Geometry: see drawing. Coordinates: mm, zero at the bounding-box minimum. A direction names the side the tool comes from. Give positions to 0.01 mm unless a question says otherwise; leave off trailing zeros. Loops run counter-clockwise (first coordinate to the right, second up) from the corner with the lowest first, then second, coordinate; pieces in that order, holes last. Notation, with made-up numbers: (-2, -5) - (45, -5) arc R14 ccw to (45, 8) - close; hole circle Ø2 at (-13, -28.75). An arc over 180 degrees is marked (long way). Use one line per item in the form item = value.
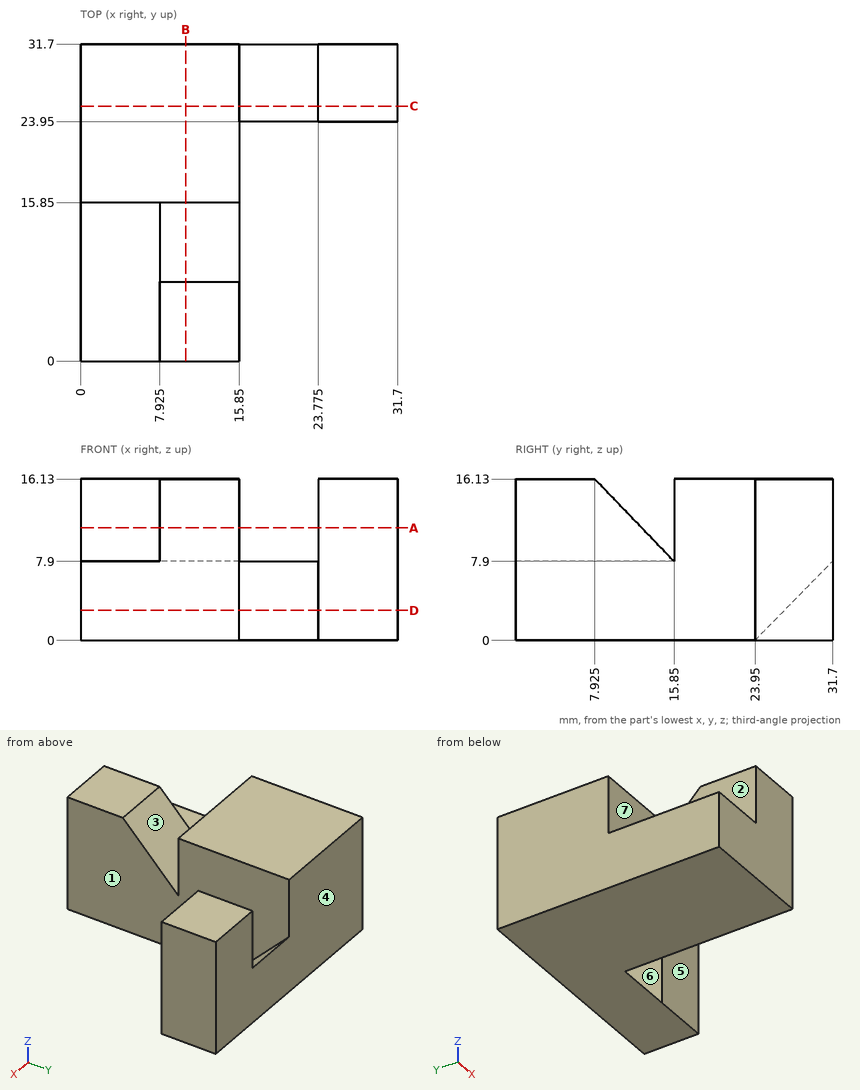
(1) Cut plane A-A (z = 11.25). Return the cut outline in (x, y) (3 decimals).
Solution:
outline = (0, 15.85) - (15.85, 15.85) - (15.85, 31.7) - (0, 31.7) - close; (7.925, 0) - (15.85, 0) - (15.85, 12.624) - (7.925, 12.624) - close; (23.775, 23.95) - (31.7, 23.95) - (31.7, 31.7) - (23.775, 31.7) - close
(2) Material intervals for L1, parallel to X at y = 24, z = 1.5 (3 decimals); L2, parallel to Y at x = 25, z = 8.5; L3, parallel to X at y = 22, z = 15.25, sorted ascending. Write a range as from..to.
Solution:
L1 = 0..15.85, 23.775..31.7
L2 = 23.95..31.7
L3 = 0..15.85
(3) Cut plane C-C (y = 25.5). Return the cut outline in (x, z) (3 decimals).
Solution:
outline = (0, 0) - (31.7, 0) - (31.7, 16.13) - (23.775, 16.13) - (23.775, 1.58) - (15.85, 1.58) - (15.85, 16.13) - (0, 16.13) - close
(4) Pin query (flat end, axial travel): P1, Ø4, axis at y = 12.5, z = 14, coming from the -X side (3 decimals); P2, Ø8, axis at y = 18.5, z = 5.5, coming from the +X side; P3, Ø4, axis at x = 28.5, z = 7.5, coming from the -Y side. Return the tip coordinate at first contact, or that it passes through.
Solution:
P1 = 7.925
P2 = 15.85
P3 = 23.95
(5) Cut plane B-B (x = 10.5). Return the cut outline in (y, z) (3 decimals), plus the area to 3 significant figures.
Solution:
outline = (0, 0) - (31.7, 0) - (31.7, 16.13) - (15.85, 16.13) - (15.85, 7.9) - (7.925, 16.13) - (0, 16.13) - close
area = 479 mm2
(6) Cut plane D-D (z = 3). Return the cut outline in (x, y) (3 decimals).
Solution:
outline = (0, 0) - (15.85, 0) - (15.85, 26.893) - (23.775, 26.893) - (23.775, 23.95) - (31.7, 23.95) - (31.7, 31.7) - (0, 31.7) - close
(7) Pull-direction query (Y, two-part tool) for the marked faces 4, 5, 6 and 7; classes: released by +Y, released by -Y, zero draft, split by the parting line, or undercut.
Solution:
face_4 = released by +Y
face_5 = released by -Y
face_6 = zero draft
face_7 = undercut
(8) Access query for the marked faces 1, 2 and 3. Directions: +Z, -Z, +X, -X, +Y, -Y. A direction counts if a zero-diameter tool reaches every point of the face in a straight line with its end or side. Return the directions, or none.
Solution:
face_1 = +Z, -Y
face_2 = +Z, -X, -Y
face_3 = +Z, +X, -X
